Could you check a few things on this model? Use its own coordinates, in mm. Face numbers are marked on the shaded views. A direction names the side the tool comes from. Coordinates: 2 decimals unless noted, no trailing zeros. Order: outer loops, then holes, each group sorted by start corner. A loop starts at its lowest first (then second) coordinate and runs counter-clockwise, first axis right, second up. Notation, with made-up numbers: M 27.5,10.5 L 51.5,10.5 A26 ccw 51.5,29.5 Z; hole C 47,89 d10. An arc over 180 degrees is marked long. Write item = value, one per line. Start each with the question number.
from build123d import *

# Parameters (mm, degrees)
SKETCH1_W           = 55
SKETCH1_H           = 20
BOSS_EXTRUDE1_DEPTH = 2
SKETCH2_W           = 2.5
SKETCH2_H           = 20
BOSS_EXTRUDE2_DEPTH = 25
SKETCH3_R           = 1.5
CUT_EXTRUDE1_DEPTH  = 3


with BuildPart() as part:
    # Sketch1 → Boss-Extrude1 (new body)
    with BuildSketch(Plane(origin=(0, 0, 0), x_dir=(1, 0, 0), z_dir=(0, 1, 0))):
        Rectangle(SKETCH1_W, SKETCH1_H)
    extrude(amount=BOSS_EXTRUDE1_DEPTH)

    # Sketch2 → Boss-Extrude2 (add)
    with BuildSketch(Plane(origin=(0, 2, 0), x_dir=(1, 0, 0), z_dir=(0, 1, 0))):
        with Locations((-26.25, 0)):
            Rectangle(SKETCH2_W, SKETCH2_H)
        with Locations((26.25, 0)):
            Rectangle(SKETCH2_W, SKETCH2_H)
    extrude(amount=BOSS_EXTRUDE2_DEPTH)

    # Sketch3 → Cut-Extrude1 (cut, through all)
    with BuildSketch(Plane(origin=(0, 2, 0), x_dir=(1, 0, 0), z_dir=(0, 1, 0))):
        with Locations((5, 5)):
            Circle(SKETCH3_R)
        with Locations((-5, 5)):
            Circle(SKETCH3_R)
        with Locations((-5, -5)):
            Circle(SKETCH3_R)
        with Locations((5, -5)):
            Circle(SKETCH3_R)
    extrude(amount=-CUT_EXTRUDE1_DEPTH, mode=Mode.SUBTRACT)


solid = part.part
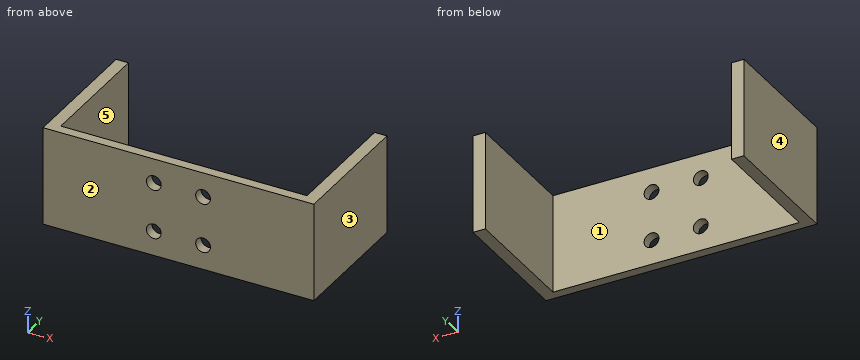
(1) Please list where these lines run through material, in increasing order: probe 1 along Z at (x, y) = (5, 0.9); probe 2 along X at (y, z) = (20.75, -0.25); probe 3 along X at (y, z) = (1.05, -5). Write a range as from..to.
(2) Will these pins go through, and if not, where does the flat tip stop? P1, Ø3.5, axis at x = 5, z = 5, coming from the +Y side; P2, Ø1.8, axis at x = 5, z = -5, coming from the +Y side; P3, Ø3, axis at x = -17, z = 0.5, coming from the -Y side.
(3) Imagine slicing it at C-C on x = -5. List the corners of the cut face in (y, z) for me.
(4) For the marked faces 4 and 5, which set-ups out of +Z, -Z, +X, -X, +Y, -Y let a thin tool reach every point of the face, with its end or its side?
(5) Imagine slicing it at A-A on z = -5. List the corners of the cut face in (x, y) for me, plus the area to 3 significant figures.
(6) Imagine slicing it at B-B on y = 11. List the corners of the cut face in (x, z) for me, plus the area to 3 significant figures.
(7) Thinking about a two-plate mould opening in X: for the marked faces 1, 2 and 3, which applies, released by +X, released by -X, zero draft, split by the parting line, or undercut?
(8) Imagine slicing it at D-D on z = 8.75. List the corners of the cut face in (x, y) for me, plus the area to 3 significant figures.
Response:
q1.probe_1 = -10..-6.5, -3.5..3.5, 6.5..10
q1.probe_2 = -27.5..-25, 25..27.5
q1.probe_3 = -27.5..-6.5, -3.5..3.5, 6.5..27.5
q2.P1 = 2
q2.P2 = through
q2.P3 = 0
q3.outline = M 0,-10 L 2,-10 L 2,-6.5 L 0,-6.5 Z; M 0,-3.5 L 2,-3.5 L 2,3.5 L 0,3.5 Z; M 0,6.5 L 2,6.5 L 2,10 L 0,10 Z
q4.face_4 = +Z, -Z, -X, +Y, -Y
q4.face_5 = +Z, -Z, +Y
q5.outline = M -27.5,0 L -6.5,0 L -6.5,2 L -25,2 L -25,27 L -27.5,27 Z; M -3.5,0 L 3.5,0 L 3.5,2 L -3.5,2 Z; M 6.5,0 L 27.5,0 L 27.5,27 L 25,27 L 25,2 L 6.5,2 Z
q5.area = 223 mm2
q6.outline = M -27.5,-10 L -25,-10 L -25,10 L -27.5,10 Z; M 25,-10 L 27.5,-10 L 27.5,10 L 25,10 Z
q6.area = 100 mm2
q7.face_1 = undercut
q7.face_2 = zero draft
q7.face_3 = released by +X
q8.outline = M -27.5,0 L 27.5,0 L 27.5,27 L 25,27 L 25,2 L -25,2 L -25,27 L -27.5,27 Z
q8.area = 235 mm2
